Here's how the part is built. I have some questions about the finished solid (model axes, mm). Face numbers are marked on the shaded views. A direction names the side the tool comes from. Round coordinates to 2 decimals unless told otherwise and drop trailing zeros. Loops run counter-clockwise (first coordinate to the right, second up) from the corner with the lowest first, then second, coordinate; pieces in that order, holes last. Notation, with made-up numbers: M 88,15.5 L 98,15.5 A19 ccw 98,20.5 Z; hole C -14.5,-39 d5. An arc over 180 degrees is marked long. Answer as a JSON object with one key per item and string values.
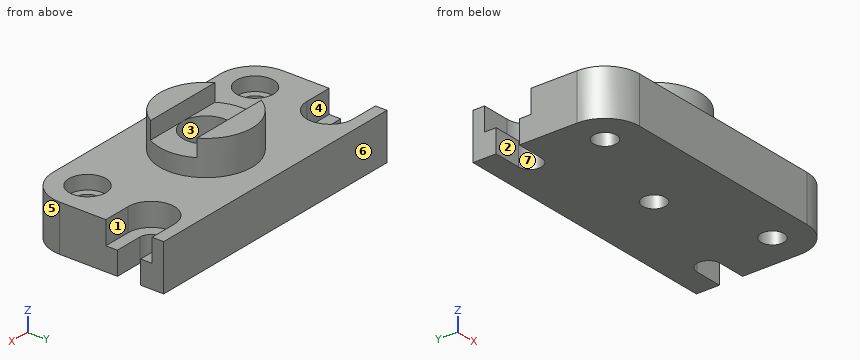
from build123d import *

# Parameters (mm, degrees)
F1_DEPTH        = 20
F2_R            = 20
F3_DEPTH        = 15
F6_DEPTH        = 20.001
F7_DEPTH        = 10
F8_D            = 10
F8_CBORE_D      = 16
F8_CBORE_DEPTH  = 6
F10_D           = 10
F10_CBORE_D     = 20
F10_CBORE_DEPTH = 25
F12_DEPTH       = 7.5


# Not quite as in the source:
# - a feature names something its author has since deleted; it is built from what else it names


with BuildPart() as f1:
    # F0 (on Top) → F1 (new body)
    with BuildSketch(Plane.XY):
        with BuildLine():
            Line((60, 30), (-60, 30))
            Line((-60, 30), (-60, -15))
            ThreePointArc((-60, -15), (-55.6066017178, -25.6066017178), (-45, -30))
            Line((-45, -30), (45, -30))
            ThreePointArc((45, -30), (55.6066017178, -25.6066017178), (60, -15))
            Line((60, -15), (60, 30))
        make_face()
    extrude(amount=F1_DEPTH)

    # F2 (on face) → F3 (join)
    with BuildSketch(Plane.XY.offset(20)):
        Circle(F2_R)
    extrude(amount=F3_DEPTH)

    # F5 (on face) → F6 (cut, through all)
    with BuildSketch(Plane.XY.offset(20)):
        with BuildLine():
            Line((-60, 20), (-60, 10))
            Line((-60, 10), (-48, 10))
            ThreePointArc((-48, 10), (-43, 15), (-48, 20))
            Line((-48, 20), (-60, 20))
        make_face()
        with BuildLine():
            Line((60, 10), (60, 20))
            Line((60, 20), (48, 20))
            ThreePointArc((48, 20), (43, 15), (48, 10))
            Line((48, 10), (60, 10))
        make_face()
    extrude(amount=-F6_DEPTH, mode=Mode.SUBTRACT)

    # F5 (on face) → F7 (cut)
    with BuildSketch(Plane.XY.offset(20)):
        with BuildLine():
            Line((-60, 5), (-48, 5))
            ThreePointArc((-48, 5), (-38, 15), (-48, 25))
            Line((-48, 25), (-60, 25))
            Line((-60, 25), (-60, 20))
            Line((-60, 20), (-48, 20))
            ThreePointArc((-48, 20), (-43, 15), (-48, 10))
            Line((-48, 10), (-60, 10))
            Line((-60, 10), (-60, 5))
        make_face()
        with BuildLine():
            Line((60, 20), (60, 25))
            Line((60, 25), (48, 25))
            ThreePointArc((48, 25), (38, 15), (48, 5))
            Line((48, 5), (60, 5))
            Line((60, 5), (60, 10))
            Line((60, 10), (48, 10))
            ThreePointArc((48, 10), (43, 15), (48, 20))
            Line((48, 20), (60, 20))
        make_face()
    extrude(amount=-F7_DEPTH, mode=Mode.SUBTRACT)

    # F8 (through all)
    with Locations(Plane.XY.offset(20)):
        with Locations((-45, -15), (45, -15)):
            CounterBoreHole(F8_D / 2, F8_CBORE_D / 2, F8_CBORE_DEPTH)

    # F10 (through all)
    with Locations(Plane.XY.offset(35)):
        with Locations((0, 0)):
            CounterBoreHole(F10_D / 2, F10_CBORE_D / 2, F10_CBORE_DEPTH)

    # F11 (on face) → F12 (cut)
    with BuildSketch(Plane.XY.offset(35)):
        with BuildLine():
            Line((-3.73e-08, 10), (-17.3205080757, 10))
            ThreePointArc((-17.3205080757, 10), (-19.3185165265, 5.1763808994), (-20, -5.5e-09))
            ThreePointArc((-20, -5.5e-09), (-19.3185165251, -5.1763809047), (-17.3205080757, -10))
            Line((-17.3205080757, -10), (0, -10))
            ThreePointArc((0, -10), (-10, -1.87e-08), (-3.73e-08, 10))
        make_face()
        with BuildLine():
            Line((17.3205080757, 10), (-3.73e-08, 10))
            ThreePointArc((-3.73e-08, 10), (7.0710677987, 7.0710678251), (10, 0))
            ThreePointArc((10, 0), (7.0710678119, -7.0710678119), (0, -10))
            Line((0, -10), (17.3205080757, -10))
            ThreePointArc((17.3205080757, -10), (19.3185165258, -5.1763809021), (20, 0))
            ThreePointArc((20, 0), (19.3185165258, 5.1763809021), (17.3205080757, 10))
        make_face()
    extrude(amount=-F12_DEPTH, mode=Mode.SUBTRACT)


solid = f1.part
Item 1: If I drill on L1, parallel to Y at x = 0, z = 20.25; L2, parallel to Y at x = 0, z = 17, over which ranges is the centre line in solid material (lowest first)? Write a range as from..to.
Solution:
{"L1": "y = -20..-10, 10..20", "L2": "y = -30..-10, 10..30"}
Item 2: I want a section at A-A on y = 0. List the corners of the cut face in (x, z) for me.
Solution:
{"outline": "M -60,0 L -5,0 L -5,10 L -10,10 L -10,27.5 L -20,27.5 L -20,20 L -60,20 Z; M 5,0 L 60,0 L 60,20 L 20,20 L 20,27.5 L 10,27.5 L 10,10 L 5,10 Z"}
Item 3: I want a section at D-D on z = 33.5. List the corners of the cut face in (x, y) for me, plus the area to 3 significant figures.
Solution:
{"outline": "M -17.32,-10 A20 ccw 17.32,-10 Z; M -17.32,10 L 17.32,10 A20 ccw Z", "area": "491 mm2"}
Item 4: For the marked faces 1, 2, 3 and 4, which set-ups out of +Z, -Z, +X, -X, +Y, -Y let a thin tool reach every point of the face, with its end or its side?
Solution:
{"face 1": "+Z, +X", "face 2": "+Z, -Z, -X", "face 3": "+Z", "face 4": "+Z, -X"}
Item 5: For P1, Ø22, axis at x = -8.5, y = -4, coming from the +Z side; P2, Ø6, axis at x = -1, z = 30.5, coming from the -Y side; P3, Ø8, axis at x = 48.5, y = -16.5, coming from the +Z side; P4, Ø10, axis at y = -19, z = 30, coming from the -X side, each with a flat end and sliding along its axis, tell me the tip position at first contact or that it passes through.
Solution:
{"P1": "stops at z = 35", "P2": "stops at y = -20", "P3": "stops at z = 14", "P4": "stops at x = -14.28"}
Item 6: I want a section at C-C on y = -12. List the corners of the cut face in (x, z) for me, plus the area to 3 significant figures.
Solution:
{"outline": "M -60,0 L -49,0 L -49,14 L -52.42,14 L -52.42,20 L -60,20 Z; M -41,0 L 41,0 L 41,14 L 37.58,14 L 37.58,20 L 16,20 L 16,35 L -16,35 L -16,20 L -37.58,20 L -37.58,14 L -41,14 Z; M 49,0 L 60,0 L 60,20 L 52.42,20 L 52.42,14 L 49,14 Z", "area": "2,480 mm2"}
Item 7: I want a section at B-B on z = 17. List the corners of the cut face in (x, y) for me, plus the area to 3 significant figures.
Solution:
{"outline": "M -60,-15 A15 ccw -45,-30 L 45,-30 A15 ccw 60,-15 L 60,5 L 48,5 A10 cw 48,25 L 60,25 L 60,30 L -60,30 L -60,25 L -48,25 A10 cw -48,5 L -60,5 Z; hole C -45,-15 d16; hole C 0,0 d20; hole C 45,-15 d16", "area": "5,590 mm2"}
Item 8: We'd pull the mould along Y, two halves only. Please class the marked faces 5, 6 and 7: +Y half, -Y half, draft (parallel to the pull), parting line (faces both ways), or undercut.
Solution:
{"face 5": "-Y half", "face 6": "+Y half", "face 7": "undercut"}
